Geometry check sheet. Reference: drawing and pictorial views, mm from the part's lowest x, y, z. A direction names the side the tool comes from. Round coordinates to 2 decimals unless told otherwise and drop trailing zeros. Write each loop counter-clockwise with the first axis right and the second up, starting at its lowest first coordinate (ties: lowest second). Pieces come first, ordered by that corner, then holes. Notation, with made-up numbers: (-9.75, 14.25) -> (35.25, 14.25) arc R25 cw to (35.25, 41.25) -> close; hole circle Ø5 at (62, 22.5). An arc over 180 degrees is marked (long way). Answer as a JSON object with one key per item and string values. Group by question number.
(1) Draft check along Y on the marked faces 3, 4 and 5. Enter one of: released by +Y, released by -Y, zero draft, split by the parting line, or undercut.
(2) Scan lines: L1, parallel to X at y = 24.15, z = 4; L2, parallel to Y at x = 15, z = 5.25; L3, parallel to Z at x = 24, y = 3. Record each from-to range of solid material in increasing order. Write a range as from..to.
(3) Sectioned sample at B-B on z = 15.75. Record the cut outline in (x, y).
(4) Set-up check for the marked faces 1 and 2: record each of +Z, -Z, +X, -X, +Y, -Y from which the full face is reachable in a straight line by a thin tool's end or side.
(5) Sectioned sample at C-C on x = 26.5. Record the cut outline in (y, z).
(6) Sectioned sample at D-D on y = 15.5. Record the cut outline in (x, z), and give its area (3 significant figures).
(7) Gauge pin test, flat ends, axial feed: pin 1 Ø5 at (y, z) = (34.5, 7.5) entering from +X; pin 2 Ø7 at (x, z) = (19.5, 8) entering from -Y; pin 3 Ø6.5 at (x, y) = (15, 24.15) entering from +Z; pin 4 Ø6 at (x, z) = (6, 16) entering from +Y. Record the tip position at first contact, or that the pin passes through.
(8) Sectioned sample at A-A on x = 15. Record the cut outline in (y, z).
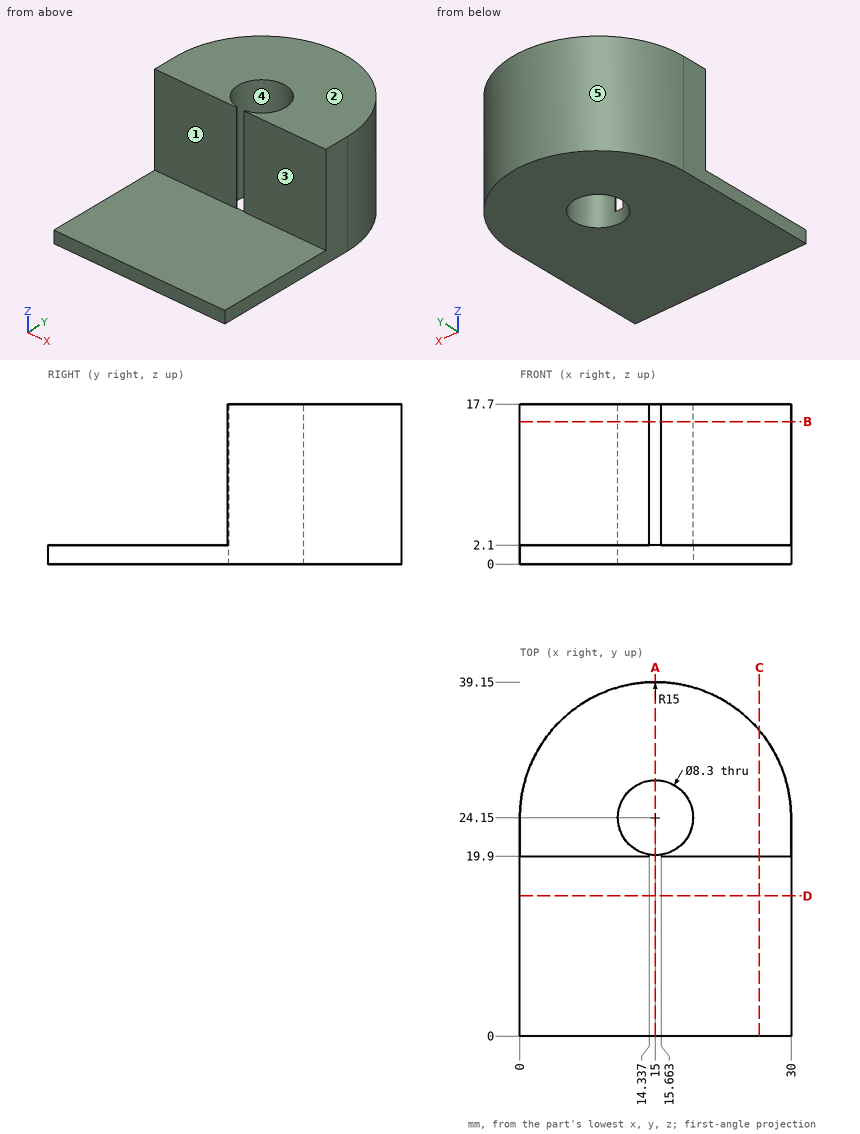
Computed values:
{
 "1": {"face 3": "released by -Y", "face 4": "undercut", "face 5": "released by +Y"},
 "2": {"L1": "0..10.85, 19.15..30", "L2": "28.3..39.15", "L3": "0..2.1"},
 "3": {"outline": "(0, 19.9) -> (14.34, 19.9) -> (14.34, 20.05) arc R4.15 cw (long way) to (15.66, 20.05) -> (15.66, 19.9) -> (30, 19.9) -> (30, 24.15) arc R15 ccw to (0, 24.15) -> close"},
 "4": {"face 1": "+Z, +X, -X, -Y", "face 2": "+Z, +X, -X, +Y, -Y"},
 "5": {"outline": "(0, 0) -> (33.78, 0) -> (33.78, 17.7) -> (19.9, 17.7) -> (19.9, 2.1) -> (0, 2.1) -> close"},
 "6": {"outline": "(0, 0) -> (30, 0) -> (30, 2.1) -> (0, 2.1) -> close", "area": "63.0 mm2"},
 "7": {"pin 1": "x = 27.78", "pin 2": "y = 19.9", "pin 3": "through", "pin 4": "y = 37.9"},
 "8": {"outline": "(0, 0) -> (20, 0) -> (20, 2.1) -> (0, 2.1) -> close; (28.3, 0) -> (39.15, 0) -> (39.15, 17.7) -> (28.3, 17.7) -> close"}
}
